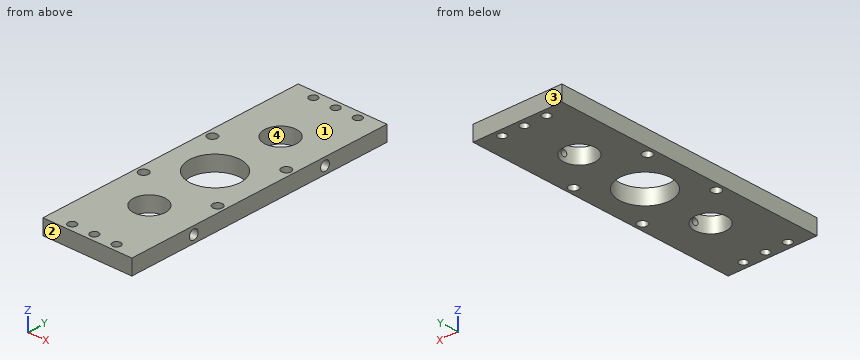
from build123d import *

# Parameters (mm, degrees)
ESBO_O1_W                = 56
ESBO_O1_H                = 173
RESSALTO_EXTRUS_O1_DEPTH = 9.525
ESBO_O2_R                = 16
ESBO_O2_R_2              = 10
ESBO_O2_R_3              = 2.6
CORTE_EXTRUS_O1_DEPTH    = 9.525
CORTAR_EXTRUIR2_REACH    = 105.484
CROQUIS1_R               = 2
CROQUIS2_R               = 3
CORTAR_EXTRUIR3_DEPTH    = 7
ESBO_O3_R                = 3
CORTE_EXTRUS_O2_DEPTH    = 92.416495376


with BuildPart() as part:
    # Esboço1 → Ressalto-extrusão1 (new body)
    with BuildSketch(Plane.XY):
        Rectangle(ESBO_O1_W, ESBO_O1_H)
    extrude(amount=RESSALTO_EXTRUS_O1_DEPTH)

    # Esboço2 → Corte-extrusão1 (cut)
    with BuildSketch(Plane.XY.offset(9.525)):
        Circle(ESBO_O2_R)
        with Locations((0, 44.47)):
            Circle(ESBO_O2_R_2)
        with Locations((0, -44.47)):
            Circle(ESBO_O2_R_2)
        with Locations((0, 81.74)):
            Circle(ESBO_O2_R_3)
        with Locations((14, 81.74)):
            Circle(ESBO_O2_R_3)
        with Locations((-14, 81.74)):
            Circle(ESBO_O2_R_3)
        with Locations((14, -81.74)):
            Circle(ESBO_O2_R_3)
        with Locations((0, -81.74)):
            Circle(ESBO_O2_R_3)
        with Locations((-14, -81.74)):
            Circle(ESBO_O2_R_3)
    extrude(amount=-CORTE_EXTRUS_O1_DEPTH, mode=Mode.SUBTRACT)

    # Croquis1 → Cortar-Extruir2 (cut, up to next)
    with BuildSketch(Plane(origin=(28, 0, 0), x_dir=(0, 0, -1), z_dir=(1, 0, 0)), mode=Mode.PRIVATE) as cortar_extruir2_sk1:
        with Locations(Location((-4.7625, -44.47, 0), (0, 0, 90))):
            Circle(CROQUIS1_R)
    cortar_extruir2_tool1 = extrude(cortar_extruir2_sk1.sketch, amount=-CORTAR_EXTRUIR2_REACH, mode=Mode.PRIVATE) & part.part
    # Croquis1 → Cortar-Extruir2 (cut, up to next)
    with BuildSketch(Plane(origin=(28, 0, 0), x_dir=(0, 0, -1), z_dir=(1, 0, 0)), mode=Mode.PRIVATE) as cortar_extruir2_sk2:
        with Locations(Location((-4.7625, 44.47, 0), (0, 0, 90))):
            Circle(CROQUIS1_R)
    cortar_extruir2_tool2 = extrude(cortar_extruir2_sk2.sketch, amount=-CORTAR_EXTRUIR2_REACH, mode=Mode.PRIVATE) & part.part
    add(cortar_extruir2_tool1.solids().sort_by_distance((28, -44.47, 4.7625))[0], mode=Mode.SUBTRACT)
    add(cortar_extruir2_tool2.solids().sort_by_distance((28, 44.47, 4.7625))[0], mode=Mode.SUBTRACT)

    # Croquis2 → Cortar-Extruir3 (cut)
    with BuildSketch(Plane(origin=(28, 0, 0), x_dir=(0, 0, -1), z_dir=(1, 0, 0))):
        with Locations(Location((-4.7625, -44.47, 0), (0, 0, 90))):
            Circle(CROQUIS2_R)
        with Locations(Location((-4.7625, 44.47, 0), (0, 0, 90))):
            Circle(CROQUIS2_R)
    extrude(amount=-CORTAR_EXTRUIR3_DEPTH, mode=Mode.SUBTRACT)

    # Esboço3 → Corte-extrusão2 (cut, through all)
    with BuildSketch(Plane.XY.offset(9.525)):
        with Locations((-23.3, 23.3)):
            Circle(ESBO_O3_R)
        with Locations((23.3, 23.3)):
            Circle(ESBO_O3_R)
        with Locations((23.3, -23.3)):
            Circle(ESBO_O3_R)
        with Locations((-23.3, -23.3)):
            Circle(ESBO_O3_R)
    extrude(amount=-CORTE_EXTRUS_O2_DEPTH, mode=Mode.SUBTRACT)


solid = part.part
For this review, take the finished solid that the model builds, in its own axes (mm). Face numbers are marked on the shaded views. Round coordinates to 2 decimals unless told otherwise and drop trailing zeros. Order: outer loops, then holes, each group sorted by start corner. A loop starts at its lowest first (then second) coordinate and runs counter-clockwise, first axis right, second up. Notation, with made-up numbers: M -11.75,46.25 L 46.25,46.25 A29 cw 46.25,70.25 Z; hole C 89.25,6.5 d2. An arc over 180 degrees is marked long. Use a Markdown table: item, result. Add a question column.
Item 1: Insertion check: pin 1 (8 mm diameter, centred on x = 23.3, y = 23.3, fed in from +Z) (3 decimals); pin 2 (3 mm diameter, centred on y = -44.47, z = 4.76, fed in from +X); pin 3 (5.5 mm diameter, centred on y = -44.47, z = 4.76, fed in from +X). Each pin has a flat end and moves straight along its axis. Give the tip position at first contact, or say it passes through.
Item 2: Add section D-D, the plane x = 23.3. Give the boundary of the cut face in (y, z) (1 decimal), then the cut area to 3 significant figures.
Item 3: Add section A-A, the plane y = -44.47. Give the boundary of the cut face in (x, z) (1 decimal), then the cut area to 3 significant figures.
Item 4: Add section C-C, the plane y = -81.74. Give the boundary of the cut face in (x, z) (3 decimals).
Item 5: Add section B-B, the plane x = -23.3. Give the boundary of the cut face in (y, z) (3 decimals).
Item 6: To check wall thickness, follow line 1 along Y through (x, z) = (0, 2.25); line 2 along Y through (x, z) = (23, 8.75); line 3 along X through (y, z) = (-23, 7.75). State the ranges of each line that lie inside material, in increasing order.
Item 7: Mouldability with a two-part tool opening along Y and no side actions: class the marked faces 1, 2, 3 and 4 as released by +Y, released by -Y, zero draft, split by the parting line, or undercut.
Geometry results:
| question | item | result |
|---|---|---|
| 1 | pin 1 | stops at z = 9.525 |
| 1 | pin 2 | stops at x = -9.89 |
| 1 | pin 3 | stops at x = 21 |
| 2 | outline | M -86.5,0 L -26.3,0 L -26.3,9.5 L -86.5,9.5 Z; M -20.3,0 L 20.3,0 L 20.3,9.5 L -20.3,9.5 Z; M 26.3,0 L 86.5,0 L 86.5,9.5 L 26.3,9.5 Z; hole C -44.5,4.8 d6; hole C 44.5,4.8 d6 |
| 2 | area | 1,480 mm² |
| 3 | outline | M -28,0 L -10,0 L -10,9.5 L -28,9.5 Z; M 10,0 L 28,0 L 28,1.8 L 21,1.8 L 21,2.8 L 10,2.8 Z; M 10,6.8 L 21,6.8 L 21,7.8 L 28,7.8 L 28,9.5 L 10,9.5 Z |
| 3 | area | 257 mm² |
| 4 | outline | M -28,0 L -16.6,0 L -16.6,9.525 L -28,9.525 Z; M -11.4,0 L -2.6,0 L -2.6,9.525 L -11.4,9.525 Z; M 2.6,0 L 11.4,0 L 11.4,9.525 L 2.6,9.525 Z; M 16.6,0 L 28,0 L 28,9.525 L 16.6,9.525 Z |
| 5 | outline | M -86.5,0 L -26.3,0 L -26.3,9.525 L -86.5,9.525 Z; M -20.3,0 L 20.3,0 L 20.3,9.525 L -20.3,9.525 Z; M 26.3,0 L 86.5,0 L 86.5,9.525 L 26.3,9.525 Z |
| 6 | line 1 | y = -86.5 to -84.34, -79.14 to -54.47, -34.47 to -16, 16 to 34.47, 54.47 to 79.14, 84.34 to 86.5 |
| 6 | line 2 | y = -86.5 to -26.28, -20.32 to 20.32, 26.28 to 86.5 |
| 6 | line 3 | x = -28 to -26.28, -20.32 to 20.32, 26.28 to 28 |
| 7 | face 1 | zero draft |
| 7 | face 2 | released by -Y |
| 7 | face 3 | released by +Y |
| 7 | face 4 | undercut |
